```python
from build123d import *

# Parameters (mm, degrees)
F1_DEPTH = 25.4


with BuildPart() as f1:
    # F0 (on Front) → F1 (new body)
    with BuildSketch(Plane.XZ):
        with BuildLine():
            ThreePointArc((3.571875, -28.350879), (21.43125, -18.900586), (28.575, 0))
            ThreePointArc((28.575, 0), (21.43125, 18.900586), (3.571875, 28.350879))
            ThreePointArc((3.571875, 28.350879), (-28.575, 0), (3.571875, -28.350879))
        make_face()
        with BuildLine():
            ThreePointArc((-13.470384, 4.7625), (0, 14.2875), (13.470384, 4.7625))
            Line((13.470384, 4.7625), (19.05, 4.7625))
            Line((19.05, 4.7625), (19.05, -4.7625))
            Line((19.05, -4.7625), (13.470384, -4.7625))
            ThreePointArc((13.470384, -4.7625), (0, -14.2875), (-13.470384, -4.7625))
            Line((-13.470384, -4.7625), (-19.05, -4.7625))
            Line((-19.05, -4.7625), (-19.05, 4.7625))
            Line((-19.05, 4.7625), (-13.470384, 4.7625))
        make_face(mode=Mode.SUBTRACT)
        with BuildLine():
            ThreePointArc((-13.470384, -4.7625), (-14.2875, 0), (-13.470384, 4.7625))
            Line((-13.470384, 4.7625), (-19.05, 4.7625))
            Line((-19.05, 4.7625), (-19.05, -4.7625))
            Line((-19.05, -4.7625), (-13.470384, -4.7625))
        make_face()
    extrude(amount=F1_DEPTH)


solid = f1.part
```
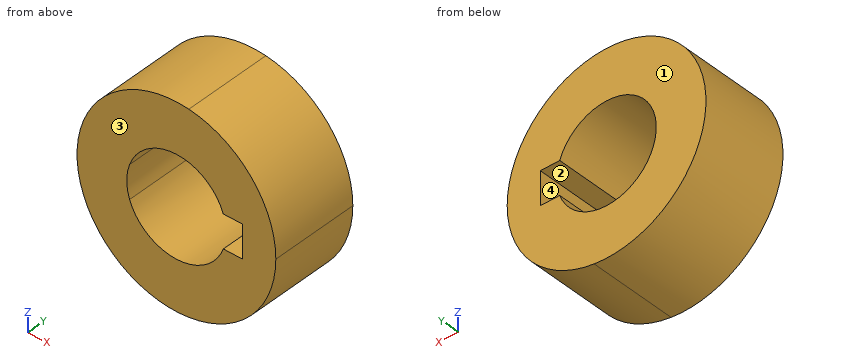
Verification items for the finished model (mm, model axes). Face numbers are marked on the shaded views. A direction names the side the tool comes from. Round coordinates to 2 decimals unless told otherwise and drop trailing zeros. Loops run counter-clockwise (first coordinate to the right, second up) from the corner with the lowest first, then second, coordinate; pieces in that order, holes last. Notation, with made-up numbers: (65, 69) -> (110, 69) arc R20 cw to (110, 103) -> close; hole circle Ø10 at (29, 27.25). An arc over 180 degrees is marked (long way). Answer as a JSON object with one key per item and string values.
Q1. Section check C-C (z = 6). Record the boundary of the cut face in (x, y), then the cut area to 3 significant figures.
Data:
{"outline": "(-27.94, -25.4) -> (-12.97, -25.4) -> (-12.97, 0) -> (-27.94, 0) -> close; (12.97, -25.4) -> (27.94, -25.4) -> (27.94, 0) -> (12.97, 0) -> close", "area": "761 mm2"}
Q2. Scan lines: line 1 (X direction, y = -5.5, z = -1); line 2 (Z direction, x = 0, y = -9) (1 decimal); line 3 (X direction, y = -8.5, z = -11). Record each from-to range of solid material in increasing order. Write a range as from..to.
Data:
{"line 1": "x = -28.56..-14.25, 19.05..28.56", "line 2": "z = -28.6..-14.3, 14.3..28.6", "line 3": "x = -26.37..-9.12, 9.12..26.37"}
Q3. Section check B-B (x = 0). Record the boundary of the cut face in (y, z) (1 decimal).
Data:
{"outline": "(-25.4, -28.6) -> (0, -28.6) -> (0, -14.3) -> (-25.4, -14.3) -> close; (-25.4, 14.3) -> (0, 14.3) -> (0, 28.6) -> (-25.4, 28.6) -> close"}
Q4. Draft check along Z on the marked faces 1 and 2. Enter one of: pulls with the +Z half, pulls with the -Z half, needs draft (parallel to the pull), parting line crosses it, or undercut.
Data:
{"face 1": "needs draft", "face 2": "undercut"}
Q5. Access from +Z, -Z, +X, -X, +Y, -Y to the whole of each face (thin tool, end or side, straight path). Record for the marked faces 3 and 4.
Data:
{"face 3": "+Z, -Z, +X, -X, -Y", "face 4": "+Y, -Y"}
Q6. Go/stop test with flat-tipped pins: P1, Ø3, axis at x = -7, y = -10.5, coming from the +Z side; P2, Ø12, axis at x = 9.5, y = -15.5, coming from the +Z side; P3, Ø6, axis at x = 17.5, y = -17.5, coming from the -Z side. Record where each tip stops, or that it passes through.
Data:
{"P1": "stops at z = 28.04", "P2": "stops at z = 28.36", "P3": "stops at z = -24.62"}
Q7. Section check D-D (x = -22.5). Record the boundary of the cut face in (y, z).
Data:
{"outline": "(-25.4, -17.61) -> (0, -17.61) -> (0, 17.61) -> (-25.4, 17.61) -> close"}
